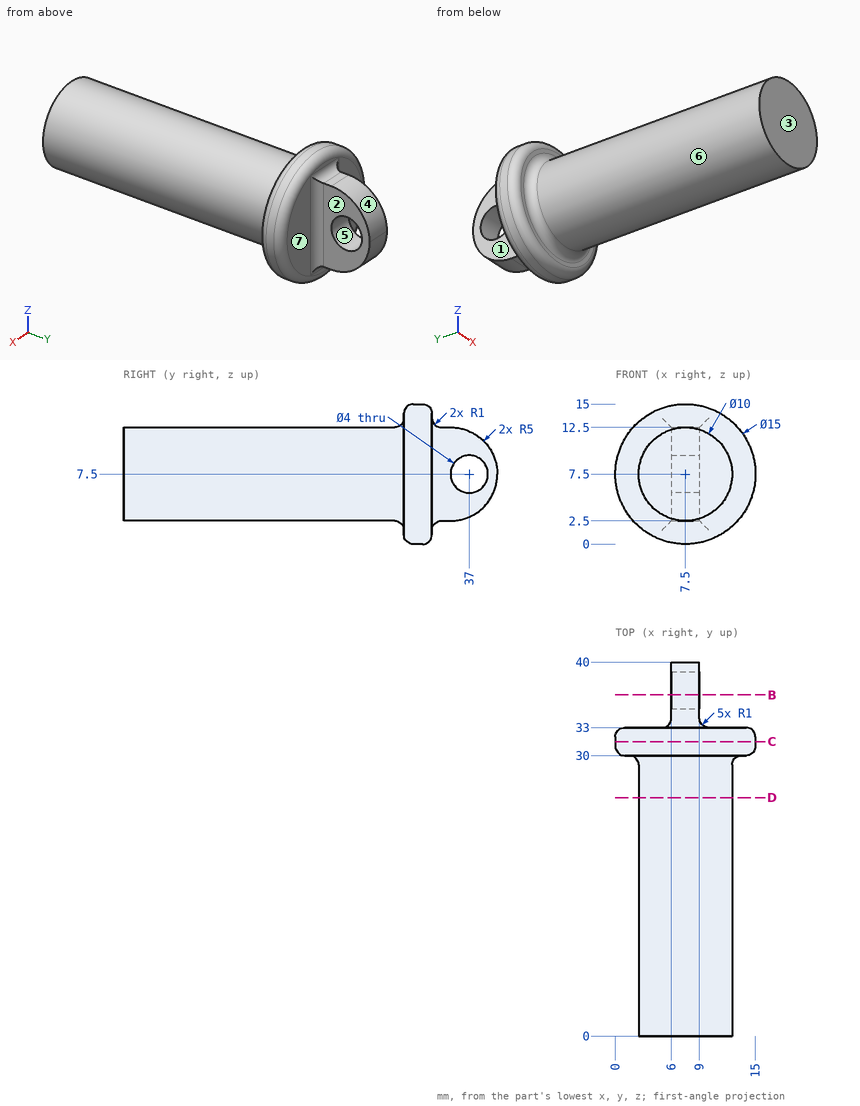
The drawing under review shows one solid part. Ordinate dimensions are in mm from its lowest x, y, z. A direction names the side the tool comes from. Round coordinates to 2 decimals unless told otherwise and drop trailing zeros. Loops run counter-clockwise (first coordinate to the right, second up) from the corner with the lowest first, then second, coordinate; pieces in that order, holes last.
Item 1: Take a section at C-C (y = 31.5). Write out the cut boundary in (x, z), then the cut area to 3 significant figures.
Determined:
outline: circle Ø15 at (7.5, 7.5)
area: 177 mm2
Item 2: Mouldability with a two-part tool opening along Z and no side actions: class the marked faces 4, 5, 6 and 7 as released by +Z, released by -Z, zero draft, split by the parting line, or undercut.
Determined:
face 4: released by +Z
face 5: undercut
face 6: split by the parting line
face 7: zero draft
Item 3: For the marked faces 1, 2 and 3, list the 3-axis set-ups (+Z, -Z, +X, -X, +Y, -Y) from which the entire face can be reached by the end or side of a thin tool; tool diameter is ignored.
Determined:
face 1: +Z, -Z, -X, +Y
face 2: +Z, -Z, +X, +Y
face 3: +Z, -Z, +X, -X, -Y
Item 4: Take a section at B-B (y = 36.5). Write out the cut boundary in (x, z).
Determined:
outline: (6, 2.73) - (9, 2.73) - (9, 5.56) - (6, 5.56) - close; (6, 9.44) - (9, 9.44) - (9, 12.27) - (6, 12.27) - close
Item 5: Take a section at D-D (y = 25.5). Write out the cut boundary in (x, z).
Determined:
outline: circle Ø10 at (7.5, 7.5)
Item 6: For line 1 (Y direction, x = 7.35, z = 7.5); line 2 (X direction, y = 8, z = 7.5); line 3 (Y direction, x = 3.5, z = 4), list the stretches that pass through material, from the lowest coordinate up.
Determined:
line 1: y = 0 to 35, 39 to 40
line 2: x = 2.5 to 12.5
line 3: y = 29.73 to 33
Item 7: Clearance check with flat-ended pins moving along their axes: pin 1 Ø3 at (x, z) = (7, 3) entering from -Y; pin 2 Ø5 at (y, z) = (15, 10.5) entering from +X (3 decimals); pin 3 Ø0.8 at (x, y) = (7, 34.5) entering from -Z; pin 4 Ø4 at (y, z) = (23, 3.5) entering from +X. State where each tip first meets the part, or that it passes through.
Determined:
pin 1: stops at y = 0
pin 2: stops at x = 12.475
pin 3: stops at z = 2.5
pin 4: stops at x = 12.08
